Autodesk Inventor part; units mm, degrees
ref_plane "YZ Plane" through (0, 0, 0) normal (1, 0, 0) x (0, 1, 0)
ref_plane "XZ Plane" through (0, 0, 0) normal (0, 1, 0) x (-1, 0, 0)
ref_plane "XY Plane" through (0, 0, 0) normal (0, 0, 1) x (1, 0, 0)
sketch "HeadplateSketch" plane through (0, 0, 0) normal (0, 0, 1) x (1, 0, 0)
  line L0 (22.2193, -2.4109) -> (25.4193, -1.6109)
  line L1 (25.4193, -1.6109) -> (25.4193, -0.0109)
  line L2 (6.3193, 0.7891) -> (3.1193, -0.0109)
  line L3 (3.1193, -1.6109) -> (3.1193, -0.0109)
  line L4 (6.3193, 0.7891) -> (22.2193, 0.7891)
  line L5 (22.2193, 0.7891) -> (25.4193, -0.0109)
  line L6 (17.1922, 9.6958) -> (17.1922, -2.4109)
  line L7 (17.1922, 9.6958) -> (18.128, 9.6958)
  line L8 (17.1922, 9.6958) -> (15.1602, 9.6958)
  line L9 (11.7996, 5.443) -> (11.7996, -2.4109)
  line L10 (21.4383, 5.5008) -> (21.4383, -2.4109)
  line L11 (21.4383, 5.5008) -> (18.128, 9.6958)
  arc A0 (15.1602, 9.6958) -> (11.7996, 5.443) centre (17.4689, 4.4173) ccw
  line L12 (3.1193, -1.6109) -> (6.3193, -2.4109)
  line L13 (6.3193, -2.4109) -> (22.2193, -2.4109)
  point P0 (11.7996, 0.7891)
  dimension "d95" = 3.2
  dimension "d102" = 1.6
  dimension "d104" = 3.2
  dimension "d106" = 0.8
  dimension "d109" = 1.6
  dimension "d110" = 3.2
  dimension "d112" = 22.3
  dimension "d113" = 15.9
extrude "拉伸1" add sketch "HeadplateSketch" along normal blind 1.27
extrude "拉伸8" add sketch "HeadplateSketch" against normal blind 1.5 contours L13 L6 L4 L10 | L4 L6 L7 L11 L10 | L13 L9 L4 L6 | L4 L9 A0 L8 L6
sketch "草图2" plane through (15.1602, 9.6958, 1.27) normal (0, 1, 0) x (1, 0, 0)
  line L0 (-3.3633, 2.0352) -> (1.9994, 0)
  arc A0 (-3.3633, 2.77) -> (6.2787, 1.2693) centre (3.7754, 16.9113) ccw
  line L1 (1.9994, 0) -> (6.2787, 0)
  line L2 (-3.3633, 2.77) -> (6.2787, 2.77)
  line L3 (2.9678, 2.77) -> (0, 2.77)
  line L4 (6.2787, 1.2693) -> (6.2787, 2.77)
  line L5 (-3.3633, 0) -> (1.9994, 0)
  line L6 (0, 0) -> (2.9678, 0)
  line L7 (2.9678, 0) -> (2.9678, 2.77)
  line L8 (-3.3633, 0) -> (-3.3633, 2.0352)
extrude "拉伸4" cut sketch "草图2" against normal up to next contours A0 L2 L7 | L7 L2 L4 A0
sketch "草图6" plane through (6.3193, -2.4109, 0) normal (0, -1, 0) x (1, 0, 0)
  line L0 (0, 0) -> (5.4803, 0)
  line L1 (0.6566, 0) -> (5.4803, -1.4987)
  line L2 (5.4803, 0) -> (5.4803, -1.4987)
  line L3 (0.6566, 0) -> (5.4803, 0)
  arc A0 (15.1197, 0.0007) -> (5.4803, -1.4987) centre (12.6164, -15.6413) ccw
  line L4 (5.4803, 0) -> (5.4803, -1.4987)
  dimension "d119" = 0
  dimension "d120" = 0
extrude "拉伸7" add sketch "草图6" against normal up to surface (3.2 mm away)
sketch "草图3" plane through (6.3193, 0.7891, 0) normal (0, 1, 0) x (1, 0, 0)
  line L0 (0, -1.27) -> (5.4803, -1.27)
  line L1 (5.4803, 0) -> (5.4803, -1.27)
  line L2 (5.4803, 0) -> (0, 0)
  line L3 (0, 0) -> (0, -1.27)
  line L4 (5.4803, -1.27) -> (16.1538, -1.27)
  line L5 (16.1538, -1.27) -> (17.1139, -1.27)
  line L6 (17.1139, -1.27) -> (17.1139, 0.0011)
extrude "拉伸9" cut sketch "草图2" against normal up to surface (8.9067 mm away) contours L0 L5 L8
sketch "草图4" plane through (0, 0, 1.27) normal (0, 0, 1) x (1, 0, 0)
  circle A0 centre (17.2686, 8.053) radius 0.825
  circle A1 centre (18.9292, 5.5008) radius 0.825
  circle A2 centre (18.9292, 2.5892) radius 0.825
  circle A3 centre (17.1095, -0.1732) radius 0.825
  line L0 (6.3193, 0.7891) -> (11.7996, 0.7891)
  line L1 (12.1356, 5.3815) -> (12.1356, 2.0023)
  line L2 (12.1356, 5.3815) -> (17.1561, 5.3815)
  line L3 (17.1561, 5.3815) -> (17.1561, 2.008)
  line L4 (17.1561, 2.008) -> (12.1356, 2.008)
  line L5 (11.7983, 4.0675) -> (12.1356, 4.0675)
  arc A4 (17.1561, 5.3815) -> (12.1356, 5.3815) centre (14.6459, 4.9584) ccw
  arc A5 (12.1356, 2.008) -> (17.1561, 2.008) centre (14.6459, 5.3033) ccw
  circle A6 centre (19.9896, -0.1732) radius 0.825
  circle A7 centre (14.1001, -0.1732) radius 0.825
  point P0 (21.4383, 5.5008)
  dimension "d121" = 0.9623
extrude "拉伸10" cut sketch "草图4" against normal through all contours L2 L3 L4 L1 | A4 L2 | L4 A5
hole "打孔7" at (18.9292, 5.5008, 1.27) at (18.9292, 2.5892, 1.27) at (17.1095, -0.1732, 1.27) at (17.2686, 8.053, 1.27) direction (0, 0, -1) diameter 1.65 end through all
hole "打孔8" at (14.1001, -0.1732, 1.27) at (19.9896, -0.1732, 1.27) direction (0, 0, -1) diameter 1.65 end through all
properties part number "JF-JM-HC0011" material "TITANIUM, 6AL-4V, ANNEALED"
Geometry: final body of the model. Coordinates: model frame, mm. A direction names the side the tool comes from. Coordinates: 2 decimals unless noted, no trailing zeros. Order: outer loops, then holes, each group sorted by start corner. A loop starts at its lowest first (then second) coordinate and runs counter-clockwise, first axis right, second up. Notation, with made-up numbers: (-23.75, 76) -> (35.25, 76) arc R27 cw to (35.25, 108) -> close; hole circle Ø2 at (-17.75, 75). An arc over 180 degrees is marked (long way). Use CSV: the item, a comma, the result in double quotes.
1) Section D-D on x = 13.75. Output: boundary loops of the cut face in (y, z).
Findings:
outline,"(-2.41, -0.67) -> (-0.92, -0.67) -> (-0.92, 1.27) -> (-2.41, 1.27) -> close; (0.57, -0.67) -> (1.26, -0.67) -> (1.26, -0.02) -> (0.79, -0.02) -> (0.79, 1.27) -> (0.57, 1.27) -> close; (7.34, -0.67) -> (8.82, -0.67) -> (8.82, -0.02) -> (7.34, -0.02) -> close"
2) Section C-C on y = 5.75. Output: boundary loops of the cut face in (x, z), then the cut area to 3 significant figures.
Findings:
outline,"(11.86, -1.47) arc R15.84 cw to (12.23, -1.29) -> (12.23, -0.6) -> (11.86, -0.74) -> close; (17.07, 0.09) arc R15.84 cw to (18.14, 0.18) -> (18.14, 1.27) -> (17.16, 1.27) -> (17.07, 1.23) -> close; (19.72, 0.18) arc R15.84 cw to (21.24, 0.03) -> (21.24, 1.27) -> (19.72, 1.27) -> close"
area,"3.23 mm^2"
3) Section B-B on z = 0.8. State how many separate pieces and enclosed holes the cut face has, then the cut area to 3 significant figures.
Findings:
separate pieces,"1"
enclosed holes,"6"
area,"89.5 mm^2"
4) Access query for faces 1 (the flat face through (15.46, 7.572, 0.625)), 2 (the flat face through (5, -1, 0)), 3 (the flat face through (14, -2.411, 1)), 4 (the cylindrical face through (15.188, 7.446, -0.027)). Directions: +Z, -Z, +X, -X, +Y, -Y. A direction counts if a zero-diameter tool reaches every point of the face in a straight line with its end or side. Return the directions, or none.
Findings:
face 1,"+Z, -X, +Y"
face 2,"-Z, -X, +Y, -Y"
face 3,"+Z, -Z, +X, -X, -Y"
face 4,"+Z, -Z"
5) Mould query, pull axis Y, two halves, no side actions, for faces 5 (the flat face through (23, -1, 0)), 6 (the flat face through (17.156, 4, 1)), 7 (the cylindrical face through (13.28, -0.07, 0.43)), 8 (the flat face through (10, 0.789, 0)). Classes: +Y half, -Y half, draft (parallel to the pull), parting line (faces both ways), or undercut.
Findings:
face 5,"draft"
face 6,"undercut"
face 7,"undercut"
face 8,"+Y half"
6) Pin query (flat end, axial travel): pin 1 Ø2 at (x, y) = (14.1, -0.17) entering from -Z; pin 2 Ø1 at (x, y) = (18.93, 2.59) entering from -Z; pin 3 Ø0.8 at (y, z) = (2.5, -1) entering from -X; pin 4 Ø3.5 at (x, y) = (22.5, -1) entering from -Z. Return the tip coordinate at first contact, or that it passes through.
Findings:
pin 1,"stops at z = -0.91"
pin 2,"passes through"
pin 3,"stops at x = 11.8"
pin 4,"stops at z = 0"
7) Line query: line 1 (X direction, y = -0.25, z = 0.25); line 2 (Y direction, x = 17.5, z = 0.45); line 3 (Y direction, x = 8.5, z = 0.45). Output: solid intervals per line, ascending.
Findings:
line 1,"x = 3.12 to 13.28, 14.92 to 16.29, 17.93 to 19.17, 20.81 to 25.42"
line 2,"y = -2.41 to -0.9, 0.55 to 7.26, 8.84 to 9.7"
line 3,"y = -2.41 to 0.79"
